Input: part model. Units: mm. Frame: model coordinates. A direction names the side the tool comes from. Coordinates: 2 decimals unless noted, no trailing zeros. Loops run counter-clockwise (first coordinate to the right, second up) from the corner with the lowest first, then second, coordinate; pieces in that order, holes last. Notation, with made-up numbers: (11, 9.5) -> (46, 9.5) arc R19 cw to (46, 15.5) -> close; hole circle Ø4 at (-10.75, 71). An arc over 180 degrees is marked (long way). Answer as a JSON object with one key per item and string values.
from build123d import *

# Parameters (mm, degrees)
F1_DEPTH = 300
F2_R     = 5
F3_R     = 2


with BuildPart() as f1:
    # F0 (on Front) → F1 (new body)
    with BuildSketch(Plane.XZ):
        Polygon((-150, 4), (-150, 0), (-30, 0), (-30, 60), (0, 60), (30, 60), (30, 0), (150, 0), (150, 4), (34, 4), (34, 64), (0, 64), (-34, 64), (-34, 4), align=None)
    extrude(amount=F1_DEPTH)

    # F2
    f2_edges = [f1.edges().sort_by_distance(p)[0] for p in [
        (-34, -150, 4),
        (34, -150, 4),
        (34, -150, 64),
        (-34, -150, 64),
    ]]
    fillet(f2_edges, radius=F2_R)

    # F3
    f3_edges = [f1.edges().sort_by_distance(p)[0] for p in [
        (30, -150, 60),
        (-30, -150, 60),
    ]]
    fillet(f3_edges, radius=F3_R)


solid = f1.part
1. Line query: line 1 along X through (y, z) = (-77, 22); line 2 along Z through (x, y) = (-70.5, -163); line 3 along Z through (x, y) = (-33, -125). Output: solid intervals per line, ascending.
Reply:
{"line 1": "x = -34 to -30, 30 to 34", "line 2": "z = 0 to 4", "line 3": "z = 0 to 62"}
2. Access query for faces 4 (the face through (95, -148, 4)), 5 (the face through (-94, -148, 4)), 6 (the face through (-30, -148, 29)), 7 (the face through (89, -148, 0)). Directions: +Z, -Z, +X, -X, +Y, -Y. A direction counts if a zero-diameter tool reaches every point of the face in a straight line with its end or side. Return the directions, or none.
Reply:
{"face 4": "+Z, +X, +Y, -Y", "face 5": "+Z, -X, +Y, -Y", "face 6": "-Z, +Y, -Y", "face 7": "-Z, +X, -X, +Y, -Y"}
3. Section query A-A (z = 34.5). Return loops of the section in (x, y), plus the area to 3 significant figures.
Reply:
{"outline": "(-34, -300) -> (-30, -300) -> (-30, 0) -> (-34, 0) -> close; (30, -300) -> (34, -300) -> (34, 0) -> (30, 0) -> close", "area": "2,400 mm2"}
4. Section query B-B (y = -112). Return loops of the section in (x, z).
Reply:
{"outline": "(-150, 0) -> (-30, 0) -> (-30, 58) arc R2 cw to (-28, 60) -> (28, 60) arc R2 cw to (30, 58) -> (30, 0) -> (150, 0) -> (150, 4) -> (39, 4) arc R5 cw to (34, 9) -> (34, 59) arc R5 ccw to (29, 64) -> (-29, 64) arc R5 ccw to (-34, 59) -> (-34, 9) arc R5 cw to (-39, 4) -> (-150, 4) -> close"}
5. Section query C-C (x = 44.5). Return loops of the section in (y, z), plus the area to 3 significant figures.
Reply:
{"outline": "(-300, 0) -> (0, 0) -> (0, 4) -> (-300, 4) -> close", "area": "1,200 mm2"}
6. Pin query (flat end, axial travel): P1, Ø5, axis at x = 21.5, y = -193.5, coming from the -Z side; P2, Ø3, axis at y = -50, z = 9.5, coming from the +X side; P3, Ø6, axis at x = -45.5, y = -54, coming from the -Z side; P4, Ø25, axis at y = -130, z = 32, coming from the +X side. Return the tip coordinate at first contact, or that it passes through.
Reply:
{"P1": "stops at z = 60", "P2": "stops at x = 34.1", "P3": "stops at z = 0", "P4": "stops at x = 34"}
7. Mould query, pull axis X, two halves, no side actions, for faces 1 (the face through (34, -148, 34)), 2 (the face through (-91, -148, 0)), 3 (the face through (0, -148, 60)). Classes: pulls with the +X half, pulls with the -X half, needs draft (parallel to the pull), parting line crosses it, or undercut.
Reply:
{"face 1": "pulls with the +X half", "face 2": "needs draft", "face 3": "undercut"}
